For this review, take the finished solid that the model builds, in its own axes (mm). Coordinates: 2 decimals unless noted, no trailing zeros. Loops run counter-clockwise (first coordinate to the right, second up) from the corner with the lowest first, then second, coordinate; pieces in that order, holes last. Notation, with made-up numbers: M 37,87 L 54,87 A30 ccw 54,126 Z; hole C -34.5,73 d5. An arc over 180 degrees is marked long. Write item = value, one per line.
from build123d import *

# Parameters (mm, degrees)
PAD_DEPTH = 0.3
FILLET_R  = 1.6


with BuildPart() as part:
    # Sketch → Pad (new body)
    with BuildSketch(Plane.XY):
        with BuildLine():
            Line((-41.6, 6), (0, 6))
            Line((0, 6), (14, 1.3))
            Line((14, 1.3), (14, -1.3))
            Line((14, -1.3), (0, -6))
            Line((0, -6), (-41.6, -6))
            ThreePointArc((-41.6, 6), (-47.600033, 0), (-41.6, -6))
        make_face()
    extrude(amount=PAD_DEPTH)

    # Fillet
    fillet_edges = [part.edges().sort_by_distance(p)[0] for p in [
        (14, -1.3, 0.15),
        (14, 1.3, 0.15),
    ]]
    fillet(fillet_edges, radius=FILLET_R)


solid = part.part
Q1. For line 1 along X through (y, z) = (-0.25, 0.2); line 2 along Y through (x, z) = (6.5, 0.2); line 3 along Y through (x, z) = (-45, 0.25), list the stretches that pass through material, from the lowest coordinate up.
Solved:
line_1 = -47.59 to 14
line_2 = -3.82 to 3.82
line_3 = -4.94 to 4.94
Q2. Add section A-A (z = 0.15). Write out the cut boundary in (x, y), and give its area (3 significant figures).
Solved:
outline = M -41.6,-6 L 0,-6 L 12.91,-1.67 A1.6 ccw 14,-0.15 L 14,0.15 A1.6 ccw 12.91,1.67 L 0,6 L -41.6,6 A6 ccw Z
area = 657 mm²
Q3. For pin 1 Ø5 at (x, y) = (-6.5, 0) entering from -Z, flat-tipped, find the tip position at first contact; note if it passes through.
Solved:
pin_1 = 0
Q4. Add section B-B (y = -4.5). Write out the cut boundary in (x, z), and give its area (3 significant figures).
Solved:
outline = M -45.57,0 L 4.47,0 L 4.47,0.3 L -45.57,0.3 Z
area = 15.0 mm²
Q5. Add section C-C (x = 3). Write out the cut boundary in (y, z).
Solved:
outline = M -4.99,0 L 4.99,0 L 4.99,0.3 L -4.99,0.3 Z
